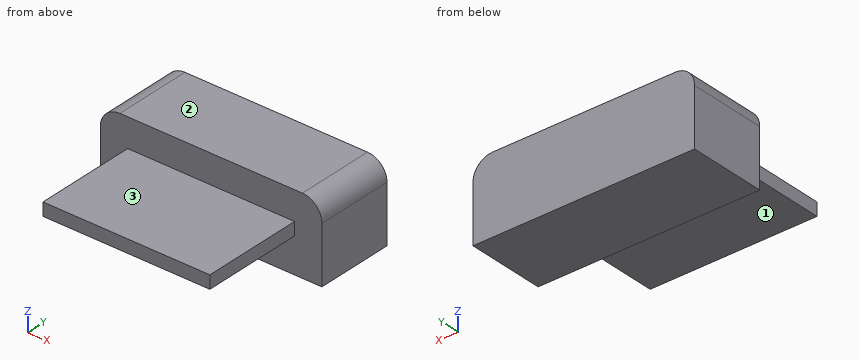
```python
from build123d import *

# Parameters (mm, degrees)
BOX001_W                  = 6.4
BOX001_H                  = 0.5
BOX001_DEPTH              = 6.9
BOX067_W                  = 8.5
BOX067_H                  = 2.95
BOX067_DEPTH              = 3
FILLET017_R               = 0.75
FUSION051_PLACEMENT_ANGLE = 90


with BuildPart() as cube043:
    # Box001 → Box001 (new body)
    with BuildSketch(Plane(origin=(-3.2, 1.35, 0), x_dir=(1, 0, 0), z_dir=(0, 0, 1))):
        with Locations((3.2, 0.25)):
            Rectangle(BOX001_W, BOX001_H)
    extrude(amount=BOX001_DEPTH)


with BuildPart() as body013:
    # Box067 → Box067 (new body)
    with BuildSketch(Plane(origin=(-4.25, 0, 0), x_dir=(1, 0, 0), z_dir=(0, 0, 1))):
        with Locations((4.25, 1.475)):
            Rectangle(BOX067_W, BOX067_H)
    extrude(amount=BOX067_DEPTH)

    # Fillet017
    fillet017_edges = [body013.edges().sort_by_distance(p)[0] for p in [
        (-4.25, 2.95, 1.5),
        (4.25, 2.95, 1.5),
    ]]
    fillet(fillet017_edges, radius=FILLET017_R)

    # Fusion051: union Cube043
    add(cube043.part)


with BuildPart() as body013_1:
    # Fusion051 placement: moved
    add(body013.part.rotate(Axis((0, 0, 0), (1, 0, 0)), FUSION051_PLACEMENT_ANGLE))


solid = body013_1.part
```
The listing builds one solid part. Answer for the finished solid, in the listing's coordinates (mm). Face numbers are marked on the shaded views. A direction names the side the tool comes from. Coordinates: 2 decimals unless noted, no trailing zeros. Loops run counter-clockwise (first coordinate to the right, second up) from the corner with the lowest first, then second, coordinate; pieces in that order, holes last. Notation, with made-up numbers: (8.5, -4) - (29.5, -4) arc R25 ccw to (29.5, 16) - close; hole circle Ø10 at (-29, -7). An arc over 180 degrees is marked (long way). Write item = value, one per line.
1) Section C-C (y = -6.25) is taken. Determine the outline of the cut face in (x, z), plus the area to 3 significant figures.
Responses:
outline = (-3.2, 1.35) - (3.2, 1.35) - (3.2, 1.85) - (-3.2, 1.85) - close
area = 3.20 mm^2
2) Section A-A (z = 1.5) is taken. Determine the outline of the cut face in (x, y), plus the area to 3 significant figures.
Responses:
outline = (-4.25, -3) - (-3.2, -3) - (-3.2, -6.9) - (3.2, -6.9) - (3.2, -3) - (4.25, -3) - (4.25, 0) - (-4.25, 0) - close
area = 50.5 mm^2
3) Section D-D (z = 0.85) is taken. Determine the outline of the cut face in (x, y), plus the area to 3 significant figures.
Responses:
outline = (-4.25, -3) - (4.25, -3) - (4.25, 0) - (-4.25, 0) - close
area = 25.5 mm^2
4) Each of these flat-tipped pins is pushed along its axis until it touches: P1, Ø1, axis at x = -1, z = 2, coming from the -Y side; P2, Ø2, axis at x = 1, y = -4.5, coming from the -Z side; P3, Ø2, axis at x = -0.5, y = -5, coming from the +Z side. Where does it stop, or does it pass through?
Responses:
P1 = -6.9
P2 = 1.35
P3 = 1.85
5) Find the intervals of material crossed by line 1 along X through (y, z) = (-3.25, 1.55); line 2 along Y through (x, z) = (-0.25, 2); line 3 along Z through (x, y) = (-1, -4.75), in increasing order.
Responses:
line_1 = -3.2 to 3.2
line_2 = -3 to 0
line_3 = 1.35 to 1.85
6) Which of the six approach directions +Z, -Z, +X, -X, +Y, -Y give full straight-line access (tool end or side, diameter ignored) to the marked faces 1, 2 and 3?
Responses:
face_1 = -Z, +X, -X, -Y
face_2 = +Z, +X, -X, +Y, -Y
face_3 = +Z, +X, -X, -Y
7) Section B-B (x = 1.5) is taken. Determine the outline of the cut face in (y, z).
Responses:
outline = (-6.9, 1.35) - (-3, 1.35) - (-3, 0) - (0, 0) - (0, 2.95) - (-3, 2.95) - (-3, 1.85) - (-6.9, 1.85) - close
